Work out the finished part from the listing and answer in its coordinate system (mm). Face numbers are marked on the shaded views. Round coordinates to 2 decimals unless told otherwise and drop trailing zeros. Loops run counter-clockwise (first coordinate to the right, second up) from the corner with the lowest first, then second, coordinate; pieces in that order, holes last.
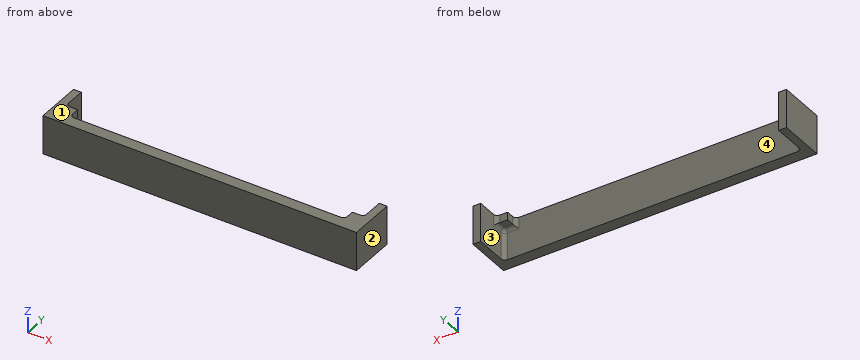
```python
from build123d import *

# Parameters (mm, degrees)
SKETCH1_W           = 81
SKETCH1_H           = 10
BOSS_EXTRUDE1_DEPTH = 3
SKETCH2_W           = 2
SKETCH2_H           = 10
BOSS_EXTRUDE2_DEPTH = 9
SKETCH3_W           = 3
SKETCH3_H           = 3
BOSS_EXTRUDE3_DEPTH = 2
FILLET1_R           = 1
FILLET2_R           = 1


with BuildPart() as part:
    # Sketch1 → Boss-Extrude1 (new body)
    with BuildSketch(Plane(origin=(0, 0, 0), x_dir=(1, 0, 0), z_dir=(0, 1, 0))):
        with Locations((40.5, 5)):
            Rectangle(SKETCH1_W, SKETCH1_H)
    extrude(amount=BOSS_EXTRUDE1_DEPTH)

    # Sketch2 → Boss-Extrude2 (add)
    with BuildSketch(Plane(origin=(0, 3, 0), x_dir=(1, 0, 0), z_dir=(0, 1, 0))):
        with Locations((1, 5)):
            Rectangle(SKETCH2_W, SKETCH2_H)
        with Locations((80, 5)):
            Rectangle(SKETCH2_W, SKETCH2_H)
    extrude(amount=BOSS_EXTRUDE2_DEPTH)

    # Sketch3 → Boss-Extrude3 (add)
    with BuildSketch(Plane.XY):
        with Locations((3.5, 4.5)):
            Rectangle(SKETCH3_W, SKETCH3_H)
        with Locations((77.5, 4.5)):
            Rectangle(SKETCH3_W, SKETCH3_H)
    extrude(amount=-BOSS_EXTRUDE3_DEPTH)

    # Fillet1
    fillet1_edges = [part.edges().sort_by_distance(p)[0] for p in [
        (79, 3, -6),
        (2, 3, -6),
    ]]
    fillet(fillet1_edges, radius=FILLET1_R)

    # Fillet2
    fillet2_edges = [part.edges().sort_by_distance(p)[0] for p in [
        (2, 5, -2),
        (2, 6, -1),
        (5, 3, -1),
        (79, 6, -1),
        (77, 3, -2),
        (76, 3, -1),
        (4, 3, -2),
        (2.292893219, 3.292893219, -2),
        (79, 5, -2),
        (78.707106781, 3.292893219, -2),
    ]]
    fillet(fillet2_edges, radius=FILLET2_R)


solid = part.part
```
1. Consider probe 1 along X at (y, z) = (9, -8.5); probe 2 along X at (y, z) = (5, -0.75); probe 3 along Y at (x, z) = (62.5, -0.75). Determine where each line is inside the solid, lowest interval first.
Answer key:
probe 1: x = 0 to 2, 79 to 81
probe 2: x = 0 to 5, 76 to 81
probe 3: y = 0 to 3
2. Given pin 1 (1 mm diameter, centred on x = 3.5, z = -1, fed in from +Y); pin 2 (1.6 mm diameter, centred on x = 77, y = 5, fed in from -Z); pin 3 (4 mm diameter, centred on x = 71, y = 6, fed in from +Z), each flat-ended and moving along its own axis, determine where each tip first touches the part or whether it passes through.
Answer key:
pin 1: stops at y = 6
pin 2: stops at z = -2
pin 3: passes through
3. Find section A-A (y = 7.75). Write down the section's boundary in (x, z).
Answer key:
outline: (0, -10) - (2, -10) - (2, 0) - (0, 0) - close; (79, -10) - (81, -10) - (81, 0) - (79, 0) - close
4. Find section C-C (x = 60). Write down the section's boundary in (y, z), then the cut area to 3 significant figures.
Answer key:
outline: (0, -10) - (3, -10) - (3, 0) - (0, 0) - close
area: 30.0 mm2
5. Find section B-B (z = -8.75). Write down the section's boundary in (x, y).
Answer key:
outline: (0, 0) - (81, 0) - (81, 12) - (79, 12) - (79, 4) arc R1 cw to (78, 3) - (3, 3) arc R1 cw to (2, 4) - (2, 12) - (0, 12) - close
6. Find section D-D (z = -1). Write down the section's boundary in (x, y), then the cut area to 3 significant figures.
Answer key:
outline: (0, 0) - (81, 0) - (81, 12) - (79, 12) - (79, 7) arc R1 cw to (78, 6) - (76, 6) - (76, 4) arc R1 cw to (75, 3) - (6, 3) arc R1 cw to (5, 4) - (5, 6) - (3, 6) arc R1 cw to (2, 7) - (2, 12) - (0, 12) - close
area: 298 mm2
7. Determine the mould class of the marked faces 1, 2, 3 and 4 for opening direction X: +X half, -X half, draft (parallel to the pull), parting line (faces both ways), or undercut.
Answer key:
face 1: draft
face 2: +X half
face 3: undercut
face 4: undercut
